from build123d import *

# Parameters (mm, degrees)
F0_R        = 2
F0_R_2      = 0.6
F1_DEPTH    = 5.35
F2_DEPTH    = 3.85
F3_T1_DEPTH = 1.5
F3_T3_DEPTH = 5.35
F3_T5_DEPTH = 8.9622341314
F3_T7_DEPTH = 4.9810546268
F3_T9_DEPTH = 5.470707469


# Not quite as in the source:
# - a fillet or chamfer that OpenCascade refuses, or shapes differently, is made with other operations: its cross-section is extruded or revolved along the edge and cut away or added


with BuildPart() as f1:
    # F0 (on Top) → F1 (new body)
    with BuildSketch(Plane.XY):
        with BuildLine():
            ThreePointArc((-2.2671417814, 1.5828117838), (-0.8296318384, -2.637600427), (2.765, 0))
            Line((2.765, 0), (5.5232667008, 3.1497960053))
            Line((5.5232667008, 3.1497960053), (3.8210715694, 6.8505014831))
            Line((3.8210715694, 6.8505014831), (1.8260751385, 7.4457344599))
            Line((1.8260751385, 7.4457344599), (-2.2671417814, 1.5828117838))
        make_face()
        Circle(F0_R, mode=Mode.SUBTRACT)
        with Locations((2.165, 6.195)):
            Circle(F0_R_2, mode=Mode.SUBTRACT)
        with BuildLine():
            Line((3.8210715694, 6.8505014831), (5.5232667008, 3.1497960053))
            Line((5.5232667008, 3.1497960053), (8.2815334016, 6.2995920106))
            ThreePointArc((8.2815334016, 6.2995920106), (6.5094775109, 12.1209007662), (0.5720401491, 13.4530626491))
            ThreePointArc((0.5720401491, 13.4530626491), (-1.0341388497, 12.8062514702), (-2.765, 12.8541613445))
            ThreePointArc((-2.765, 12.8541613445), (-3.6292192652, 11.8541613445), (-2.765, 10.8541613445))
            ThreePointArc((-2.765, 10.8541613445), (-0.9627220535, 10.7761212346), (0.7094162112, 11.4530626491))
            ThreePointArc((0.7094162112, 11.4530626491), (4.1711880344, 11.0946407177), (6.6333355769, 8.6349334352))
            ThreePointArc((6.6333355769, 8.6349334352), (6.6911609557, 7.2849011256), (5.8160680002, 6.2552685064))
            Line((5.8160680002, 6.2552685064), (3.8210715694, 6.8505014831))
        make_face()
    extrude(amount=F1_DEPTH)

    # F0 (on Top) → F2 (cut)
    with BuildSketch(Plane.XY):
        with BuildLine():
            Line((3.8210715694, 6.8505014831), (5.5232667008, 3.1497960053))
            Line((5.5232667008, 3.1497960053), (8.2815334016, 6.2995920106))
            ThreePointArc((8.2815334016, 6.2995920106), (6.5094775109, 12.1209007662), (0.5720401491, 13.4530626491))
            ThreePointArc((0.5720401491, 13.4530626491), (-1.0341388497, 12.8062514702), (-2.765, 12.8541613445))
            ThreePointArc((-2.765, 12.8541613445), (-3.6292192652, 11.8541613445), (-2.765, 10.8541613445))
            ThreePointArc((-2.765, 10.8541613445), (-0.9627220535, 10.7761212346), (0.7094162112, 11.4530626491))
            ThreePointArc((0.7094162112, 11.4530626491), (4.1711880344, 11.0946407177), (6.6333355769, 8.6349334352))
            ThreePointArc((6.6333355769, 8.6349334352), (6.6911609557, 7.2849011256), (5.8160680002, 6.2552685064))
            Line((5.8160680002, 6.2552685064), (3.8210715694, 6.8505014831))
        make_face()
    extrude(amount=F2_DEPTH, mode=Mode.SUBTRACT)

    # F3: fillet of radius 1 on 5 edges, made by hand

    # F3_s2 → F3_t1 (join)
    with BuildSketch(Plane.XY.offset(3.85)):
        with BuildLine():
            ThreePointArc((5.3238056204, 6.4021413514), (5.9123715372, 6.4072989523), (6.3960858458, 6.7426449035))
            ThreePointArc((6.3960858458, 6.7426449035), (6.1312771268, 6.4689663976), (5.8160680002, 6.2552685064))
            Line((5.8160680002, 6.2552685064), (5.3238056204, 6.4021413514))
        make_face()
    extrude(amount=F3_T1_DEPTH)

    # F3_s4 → F3_t3 (join)
    with BuildSketch(Plane.XY):
        with BuildLine():
            ThreePointArc((2.7493247705, -0.294003922), (2.8276858836, 0.0009129267), (2.9913388108, 0.258467059))
            Line((2.9913388108, 0.258467059), (2.765, 0))
            ThreePointArc((2.765, 0), (2.7610784116, -0.1472107494), (2.7493247705, -0.294003922))
        make_face()
    extrude(amount=F3_T3_DEPTH)

    # F3_s6 → F3_t5 (cut)
    with BuildSketch(Plane.XY.offset(-1.8061170657)):
        with BuildLine():
            ThreePointArc((1.41251371, 6.8533694021), (1.9030466902, 7.2251109605), (2.5183648424, 7.2391808767))
            Line((2.5183648424, 7.2391808767), (1.8260751385, 7.4457344599))
            Line((1.8260751385, 7.4457344599), (1.41251371, 6.8533694021))
        make_face()
    extrude(amount=F3_T5_DEPTH, mode=Mode.SUBTRACT)

    # F3_s8 → F3_t7 (cut)
    with BuildSketch(Plane.XY.offset(-1.1310546268)):
        with BuildLine():
            ThreePointArc((3.3875351793, 6.9798526699), (3.757108564, 6.7768067273), (4.010129337, 6.4394750953))
            Line((4.010129337, 6.4394750953), (3.8210715694, 6.8505014831))
            Line((3.8210715694, 6.8505014831), (3.3875351793, 6.9798526699))
        make_face()
    extrude(amount=F3_T7_DEPTH, mode=Mode.SUBTRACT)

    # F3_s10 → F3_t9 (cut)
    with BuildSketch(Plane.XY.offset(-1.620707469)):
        with BuildLine():
            ThreePointArc((5.2523626005, 3.738762728), (5.3335017603, 3.1773237272), (5.0961768875, 2.6620818233))
            Line((5.0961768875, 2.6620818233), (5.5232667008, 3.1497960053))
            Line((5.5232667008, 3.1497960053), (5.2523626005, 3.738762728))
        make_face()
    extrude(amount=F3_T9_DEPTH, mode=Mode.SUBTRACT)


solid = f1.part
Read the model definition and answer for the solid it produces. Units are mm, in the model's axes. A direction names the side the tool comes from. Coordinates: 2 decimals unless noted, no trailing zeros. Order: outer loops, then holes, each group sorted by start corner. A loop starts at its lowest first (then second) coordinate and runs counter-clockwise, first axis right, second up. Notation, with made-up numbers: M 5.5,22 L 63.5,22 A16 ccw 63.5,35 Z; hole C 29,-12 d8. An arc over 180 degrees is marked long. Put each result on its own line as item: value. Start each with the question number.
Item 1: For faces 1 (the face through (-0.402, 4.255, 2.638)), 2 (the face through (5.904, 6.405, 4.59)), 3 (the face through (4.62, 5.11, 1.9)), determine the directions among +Z, -Z, +X, -X, +Y, -Y from which every point of the face is accessible in a straight line to the end or side of a thin tool.
Item 2: Section A-A, the plane x = 0 is taken. Determine the outline of the cut face in (y, z) (3 decimals).
Item 3: Section B-B, the plane y = 0 is taken. Determine the outline of the cut face in (x, z) (3 decimals), plus the area to 3 significant figures.
Item 4: Consider probe 1 along Z at (x, y) = (3.5, 11.75); probe 2 along Y at (x, z) = (0, 4.2) (3 decimals); probe 3 along Y at (x, z) = (0.75, 4.5). Determine where each line is inside the solid, lowest interval first. Write a range as [from, to].
Item 5: Section D-D, the plane z = 4.55 is taken. Determine the outline of the cut face in (x, y) (1 decimal), plus the area to 3 significant figures.
Item 6: Section C-C, the plane z = 2.4 is taken. Determine the outline of the cut face in (x, y) (3 decimals), plus the area to 3 significant figures.
Item 7: Given pin 1 Ø2 at (x, z) = (-2, 1) entering from +Y; pin 2 Ø2 at (y, z) = (0, 1.5) entering from +X; pin 3 Ø2 at (y, z) = (0.5, 4.5) entering from -X (3 decimals), each flat-ended and moving along its own axis, determine where each tip first touches the part or whether it passes through.
Item 8: The mould has two halves that part along X. Classify faces 4 (the face through (4.126, 11.116, 4.59)), 5 (the face through (5.335, 3.185, 1.898)), 6 (the face through (-3.63, 11.87, 4.59)): +X half, -X half, draft (parallel to the pull), parting line (faces both ways), or undercut.
Computed:
1. face 1: +Z, -Z, -X
1. face 2: +Z, -Z
1. face 3: -Z, +X, +Y
2. outline: M -2.765,0 L -2,0 L -2,5.35 L -2.765,5.35 Z; M 2,0 L 4.83,0 L 4.83,5.35 L 2,5.35 Z; M 11.063,3.85 L 13.132,3.85 L 13.132,5.35 L 11.063,5.35 Z
3. outline: M -2.765,0 L -2,0 L -2,5.35 L -2.765,5.35 Z; M 2,0 L 2.827,0 L 2.827,5.35 L 2,5.35 Z
3. area: 8.52 mm2
4. probe 1: z = [3.85, 5.35]
4. probe 2: y = [-2.765, -2], [2, 4.83], [11.063, 13.132]
4. probe 3: y = [-2.66, -1.85], [1.85, 5.9], [11.46, 13.51]
5. outline: M -2.8,10.9 A4.2 ccw 0.7,11.5 A5.2 cw 6.6,8.6 A1.9 cw 6.4,6.7 A1 cw 5.3,6.4 L 2.5,7.2 A1 ccw 1.4,6.9 L -2.3,1.6 A2.8 ccw long 2.7,-0.3 A1 cw 3,0.3 L 8.3,6.3 A6 ccw 0.6,13.5 A4.2 cw -2.8,12.9 A1 ccw Z; hole C 0,0 d4; hole C 2.2,6.2 d1.2
5. area: 73.3 mm2
6. outline: M -2.267,1.583 A2.765 ccw long 2.749,-0.294 A1 cw 2.991,0.258 L 5.096,2.662 A1 ccw 5.252,3.739 L 4.01,6.439 A1 ccw 3.388,6.98 L 2.518,7.239 A1 ccw 1.413,6.853 Z; hole C 0,0 d4; hole C 2.165,6.195 d1.2
6. area: 35.6 mm2
7. pin 1: stops at y = 3.4
7. pin 2: stops at x = 3.64
7. pin 3: stops at x = -2.765
8. face 4: undercut
8. face 5: +X half
8. face 6: -X half
